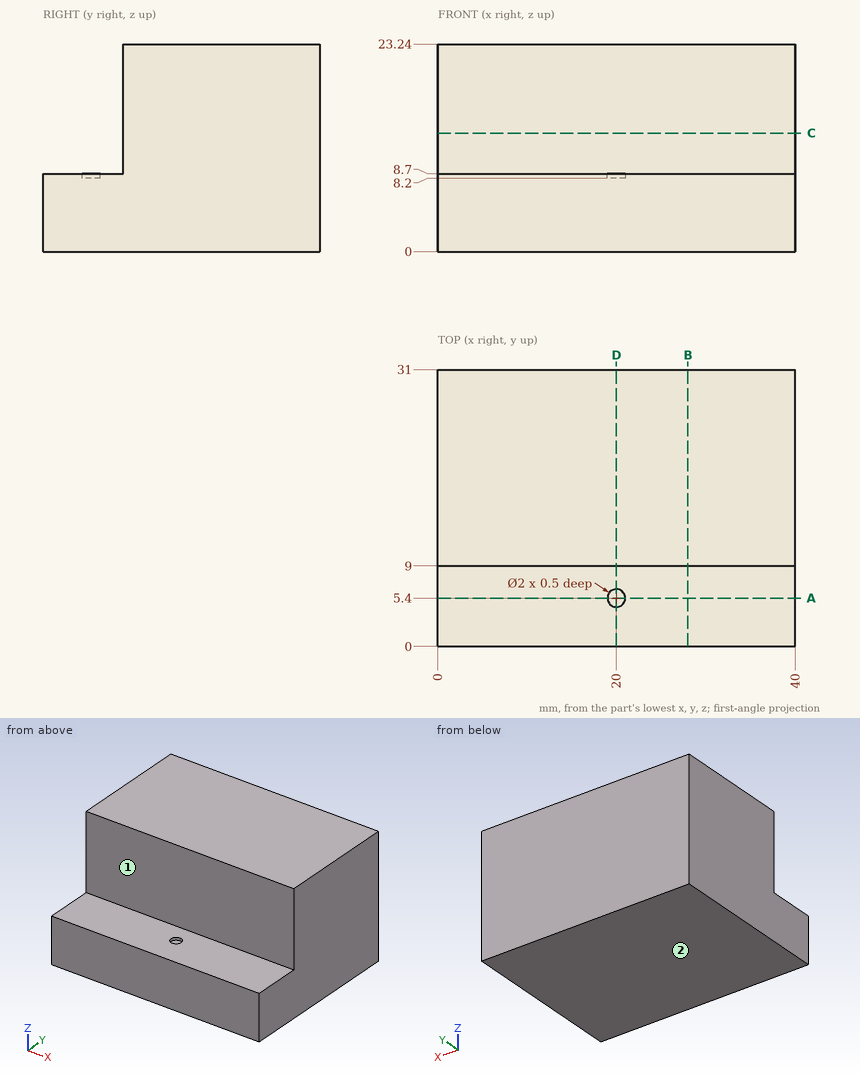
Study the drawing (mm; zero at the part's minimum x, y, z) and answer. A direction names the side the tool comes from. Coordinates: 2 decimals unless noted, no trailing zeros. Loops run counter-clockwise (first coordinate to the right, second up) from the corner with the lowest first, then second, coordinate; pieces in that order, holes last. Notation, with made-up numbers: M 77.5,-21.5 L 107.5,-21.5 A26 ccw 107.5,-6.5 Z; hole C 84,19.25 d10. An arc over 180 degrees is marked long. Answer as a JSON object with one key per item and string values. Group by question number.
Item 1: Section C-C (z = 13.25) is taken. Write down the section's boundary in (x, y), and give its area (3 significant figures).
Item 2: Section B-B (x = 28) is taken. Write down the section's boundary in (y, z).
Item 3: Consider L1, parallel to Y at x = 20, z = 8.65; L2, parallel to Z at x = 37.5, y = 1.5; L3, parallel to Y at x = 17.5, z = 13.25. Determine where each line is inside the solid, lowest interval first.
Item 4: Section D-D (x = 20) is taken. Write down the section's boundary in (y, z), and give its area (3 significant figures).
Item 5: Each of these flat-tipped pins is pushed along its axis until it touches: P1, Ø3, axis at x = 19, z = 17.5, coming from the -Y side; P2, Ø1.6, axis at x = 20, y = 5, coming from the +Z side. Where does it stop, or does it pass through?
Item 6: Section A-A (y = 5.4) is taken. Write down the section's boundary in (x, z), and give its area (3 significant figures).
Item 7: Which of the six approach directions +Z, -Z, +X, -X, +Y, -Y give full straight-line access (tool end or side, diameter ignored) to the marked faces 1 and 2?
Solved:
{
 "1": {"outline": "M 0,9 L 40,9 L 40,31 L 0,31 Z", "area": "880 mm2"},
 "2": {"outline": "M 0,0 L 31,0 L 31,23.24 L 9,23.24 L 9,8.7 L 0,8.7 Z"},
 "3": {"L1": "y = 0 to 4.4, 6.4 to 31", "L2": "z = 0 to 8.7", "L3": "y = 9 to 31"},
 "4": {"outline": "M 0,0 L 31,0 L 31,23.24 L 9,23.24 L 9,8.7 L 6.4,8.7 L 6.4,8.2 L 4.4,8.2 L 4.4,8.7 L 0,8.7 Z", "area": "589 mm2"},
 "5": {"P1": "stops at y = 9", "P2": "stops at z = 8.7"},
 "6": {"outline": "M 0,0 L 40,0 L 40,8.7 L 21,8.7 L 21,8.2 L 19,8.2 L 19,8.7 L 0,8.7 Z", "area": "347 mm2"},
 "7": {"face 1": "+Z, +X, -X, -Y", "face 2": "-Z, +X, -X, +Y, -Y"}
}
